```python
from build123d import *

# Parameters (mm, degrees)
F1_DEPTH = 19.05
F2_W     = 19.05
F2_H     = 19.05
F3_DEPTH = 19.05


with BuildPart() as f1:
    # F0 (on Top) → F1 (new body)
    with BuildSketch(Plane.XY):
        Polygon((0, 38.1), (0, 0), (19.05, 0), (19.05, 19.05), (38.1, 19.05), (38.1, 38.1), align=None)
    extrude(amount=F1_DEPTH)

    # F2 (on face) → F3 (join)
    with BuildSketch(Plane(origin=(0, 0, 0), x_dir=(1, 0, 0), z_dir=(0, 0, -1))):
        with Locations((28.575, -28.575)):
            Rectangle(F2_W, F2_H)
    extrude(amount=F3_DEPTH)


solid = f1.part
```
CAD build for the part. Positions are in the model's coordinates, mm. A direction names the side the tool comes from. Coordinates: 2 decimals unless noted, no trailing zeros. Order: outer loops, then holes, each group sorted by start corner. A loop starts at its lowest first (then second) coordinate and runs counter-clockwise, first axis right, second up. Notation, with made-up numbers: (62, 37) -> (87, 37) arc R20 cw to (87, 48) -> close; hole circle Ø6 at (87, 47). An arc over 180 degrees is marked (long way). Use one line per item in the form item = value. Start each with the question number.
1) Tool access for faces 1 (the flat face through (28, 19.05, 0)), 2 (the flat face through (38.1, 29, 0)), 3 (the flat face through (19.05, 29, -9)): list every direction of +Z, -Z, +X, -X, +Y, -Y with a clear straight run to the whole face (end or side of a thin tool).
2) Band-saw the part on C-C on x = 34. Give the cut face in (y, z), then the cut area to 3 significant figures.
3) Band-saw the part on A-A on y = 33.5. Give the cut face in (x, z).
4) Drop flat-ended pins along their axis: pin 1 (15 mm diameter, centred on y = 11, z = 11, fed in from +X); pin 2 (5.5 mm diameter, centred on x = 11.5, y = 21.5, fed in from -Z); pin 3 (15 mm diameter, centred on x = 32, z = 3.5, fed in from -Y). Give the stop position or say it passes through.
5) Drill centre lines: L1, parallel to Z at x = 18.5, y = 12; L2, parallel to Y at x = 30.5, z = -10.5. Where is each one in solid material? Low to high. Write a range as [from, to].
6) Band-saw the part on B-B on z = -1. Give the cut face in (x, y), then the cut area to 3 significant figures.
Entries:
q1.face_1 = +Z, -Z, +X, -Y
q1.face_2 = +Z, -Z, +X, +Y, -Y
q1.face_3 = -Z, -X, +Y, -Y
q2.outline = (19.05, -19.05) -> (38.1, -19.05) -> (38.1, 19.05) -> (19.05, 19.05) -> close
q2.area = 726 mm2
q3.outline = (0, 0) -> (19.05, 0) -> (19.05, -19.05) -> (38.1, -19.05) -> (38.1, 19.05) -> (0, 19.05) -> close
q4.pin_1 = 19.05
q4.pin_2 = 0
q4.pin_3 = 19.05
q5.L1 = [0, 19.05]
q5.L2 = [19.05, 38.1]
q6.outline = (19.05, 19.05) -> (38.1, 19.05) -> (38.1, 38.1) -> (19.05, 38.1) -> close
q6.area = 363 mm2
